```python
from build123d import *

# Parameters (mm, degrees)
F1_R     = 11.980735
F2_DEPTH = 23
F0_R     = 28.575
F0_R_2   = 2.54
F3_DEPTH = 4


with BuildPart() as f2:
    # F1 (on Front) → F2 (new body)
    with BuildSketch(Plane.XZ):
        with Locations((-0.001662, -0.397164)):
            Circle(F1_R)
        with BuildLine():
            add(Edge.make_bspline(
                [(2.011906, 7.609146), (2.011906, 7.809895), (2.011906, 8.211393), (2.011906, 8.813639), (2.011906, 9.215137), (2.011906, 9.415886)],
                knots=[0, 0, 0, 0, 0.602247, 1.204493, 1.80674, 1.80674, 1.80674, 1.80674], degree=3))
            ThreePointArc((2.011906, 7.609146), (4.126154, 6.752423), (5.925221, 5.349793))
            add(Edge.make_bspline(
                [(7.489904, 6.253163), (7.316434, 6.15301), (6.969194, 5.952531), (6.447633, 5.651408), (6.099543, 5.450437), (5.925221, 5.349793)],
                knots=[0, 0, 0, 0, 0.600918, 1.202873, 1.80674, 1.80674, 1.80674, 1.80674], degree=3))
            ThreePointArc((7.489904, 6.253163), (8.673752, 4.611589), (9.503473, 2.765559))
            add(Edge.make_bspline(
                [(7.93879, 1.862189), (8.113111, 1.962834), (8.461202, 2.163804), (8.982763, 2.464927), (9.330002, 2.665406), (9.503473, 2.765559)],
                knots=[0, 0, 0, 0, 0.603867, 1.205822, 1.80674, 1.80674, 1.80674, 1.80674], degree=3))
            ThreePointArc((7.93879, 1.862189), (8.25397, -0.397164), (7.93879, -2.656517))
            add(Edge.make_bspline(
                [(9.503473, -3.559887), (9.330002, -3.459734), (8.982763, -3.259255), (8.461202, -2.958132), (8.113111, -2.757162), (7.93879, -2.656517)],
                knots=[0, 0, 0, 0, 0.600918, 1.202873, 1.80674, 1.80674, 1.80674, 1.80674], degree=3))
            ThreePointArc((9.503473, -3.559887), (8.673752, -5.405917), (7.489904, -7.047491))
            add(Edge.make_bspline(
                [(5.925221, -6.144121), (6.099543, -6.244765), (6.447633, -6.445736), (6.969194, -6.746859), (7.316434, -6.947338), (7.489904, -7.047491)],
                knots=[0, 0, 0, 0, 0.603867, 1.205822, 1.80674, 1.80674, 1.80674, 1.80674], degree=3))
            ThreePointArc((5.925221, -6.144121), (4.126154, -7.546751), (2.011906, -8.403474))
            add(Edge.make_bspline(
                [(2.011906, -10.210214), (2.011906, -10.009465), (2.011906, -9.607967), (2.011906, -9.005721), (2.011906, -8.604223), (2.011906, -8.403474)],
                knots=[0, 0, 0, 0, 0.602247, 1.204493, 1.80674, 1.80674, 1.80674, 1.80674], degree=3))
            ThreePointArc((2.011906, -10.210214), (-0.001662, -10.414669), (-2.015231, -10.210214))
            add(Edge.make_bspline(
                [(-2.015231, -8.403474), (-2.015231, -8.604223), (-2.015231, -9.005721), (-2.015231, -9.607967), (-2.015231, -10.009465), (-2.015231, -10.210214)],
                knots=[0, 0, 0, 0, 0.602247, 1.204493, 1.80674, 1.80674, 1.80674, 1.80674], degree=3))
            ThreePointArc((-2.015231, -8.403474), (-4.129479, -7.546751), (-5.928546, -6.144121))
            add(Edge.make_bspline(
                [(-7.493228, -7.047491), (-7.319758, -6.947338), (-6.972519, -6.746859), (-6.450958, -6.445736), (-6.102867, -6.244765), (-5.928546, -6.144121)],
                knots=[0, 0, 0, 0, 0.600918, 1.202873, 1.80674, 1.80674, 1.80674, 1.80674], degree=3))
            ThreePointArc((-7.493228, -7.047491), (-8.677076, -5.405917), (-9.506797, -3.559887))
            add(Edge.make_bspline(
                [(-7.942115, -2.656517), (-8.116436, -2.757162), (-8.464527, -2.958132), (-8.986088, -3.259255), (-9.333327, -3.459734), (-9.506797, -3.559887)],
                knots=[0, 0, 0, 0, 0.603867, 1.205822, 1.80674, 1.80674, 1.80674, 1.80674], degree=3))
            ThreePointArc((-7.942115, -2.656517), (-8.257295, -0.397164), (-7.942115, 1.862189))
            add(Edge.make_bspline(
                [(-9.506797, 2.765559), (-9.333327, 2.665406), (-8.986088, 2.464927), (-8.464527, 2.163804), (-8.116436, 1.962834), (-7.942115, 1.862189)],
                knots=[0, 0, 0, 0, 0.600918, 1.202873, 1.80674, 1.80674, 1.80674, 1.80674], degree=3))
            ThreePointArc((-9.506797, 2.765559), (-8.677076, 4.611589), (-7.493228, 6.253163))
            add(Edge.make_bspline(
                [(-5.928546, 5.349793), (-6.102867, 5.450437), (-6.450958, 5.651408), (-6.972519, 5.952531), (-7.319758, 6.15301), (-7.493228, 6.253163)],
                knots=[0, 0, 0, 0, 0.603867, 1.205822, 1.80674, 1.80674, 1.80674, 1.80674], degree=3))
            ThreePointArc((-5.928546, 5.349793), (-4.129479, 6.752423), (-2.015231, 7.609146))
            add(Edge.make_bspline(
                [(-2.015231, 9.415886), (-2.015231, 9.215137), (-2.015231, 8.813639), (-2.015231, 8.211393), (-2.015231, 7.809895), (-2.015231, 7.609146)],
                knots=[0, 0, 0, 0, 0.602247, 1.204493, 1.80674, 1.80674, 1.80674, 1.80674], degree=3))
            ThreePointArc((-2.015231, 9.415886), (-0.001662, 9.620341), (2.011906, 9.415886))
        make_face(mode=Mode.SUBTRACT)
    extrude(amount=F2_DEPTH)

    # F0 (on Front) → F3 (join)
    with BuildSketch(Plane.XZ):
        Circle(F0_R)
        with Locations((-12.036908, -20.535689)):
            Circle(F0_R_2, mode=Mode.SUBTRACT)
        with Locations((11.767376, -20.535689)):
            Circle(F0_R_2, mode=Mode.SUBTRACT)
        with Locations((-23.8, 0)):
            Circle(F0_R_2, mode=Mode.SUBTRACT)
        with Locations((-11.988438, 20.600075)):
            Circle(F0_R_2, mode=Mode.SUBTRACT)
        with Locations((23.8, 0)):
            Circle(F0_R_2, mode=Mode.SUBTRACT)
        with Locations((11.78722, 20.636372)):
            Circle(F0_R_2, mode=Mode.SUBTRACT)
    extrude(amount=F3_DEPTH)


solid = f2.part
```
Work out the finished part from the listing and answer in its coordinate system (mm). A direction names the side the tool comes from. Coordinates: 2 decimals unless noted, no trailing zeros. Order: outer loops, then holes, each group sorted by start corner. A loop starts at its lowest first (then second) coordinate and runs counter-clockwise, first axis right, second up. Notation, with made-up numbers: (42, -37.75) - (98, -37.75) arc R21 cw to (98, -6.75) - close; hole circle Ø11 at (48.5, 75.5). An arc over 180 degrees is marked (long way). Answer as a JSON object with one key per item and string values.
1. The mould has two halves that part along Z. Classify faces 1 (the face through (0, 0, 0)), 2 (the face through (-28.547, -1.972, 1.256)), 3 (the face through (-9.566, -1.972, 21.363)): +Z half, -Z half, draft (parallel to the pull), parting line (faces both ways), or undercut.
Output values:
{"face 1": "draft", "face 2": "parting line", "face 3": "undercut"}
2. Consider line 1 (Z direction, x = 23.8, y = -2.55); line 2 (Y direction, x = 16.5, z = 22.5); line 3 (X direction, y = -18.75, z = 2). Determine where each line is inside the solid, lowest interval first.
Output values:
{"line 1": "z = -15.81 to -2.54, 2.54 to 15.81", "line 2": "y = -4 to 0", "line 3": "x = -11.74 to -8.18, 8.18 to 11.74"}
3. A tool of negligible diameter and unlimited length cuts with its end or side. For faces 4 (the face through (4.154, -13.367, -7.531)), 5 (the face through (-14.053, -1.972, -22.081)), from which of +Z, -Z, +X, -X, +Y, -Y can it reach the whole face along a straight path? Write none if from no direction.
Output values:
{"face 4": "-Y", "face 5": "+Y, -Y"}
4. Each of these flat-tipped pins is pushed along its axis until it touches: P1, Ø4.5, axis at x = 11.77, z = -20.54, coming from the +Y side; P2, Ø12, axis at x = -21.5, y = -9, coming from the +Z side; P3, Ø4, axis at x = 13.5, z = 18.5, coming from the +Y side; P4, Ø8, axis at x = -3.5, y = -6.5, coming from the -Z side. Where does it stop, or does it pass through?
Output values:
{"P1": "passes through", "P2": "stops at z = 22.04", "P3": "stops at y = 0", "P4": "stops at z = -28.57"}
5. Find section A-A on x = 23.8. Determine the outline of the cut face in (y, z), plus the area to 3 significant figures.
Output values:
{"outline": "(-4, -15.81) - (0, -15.81) - (0, -2.54) - (-4, -2.54) - close; (-4, 2.54) - (0, 2.54) - (0, 15.81) - (-4, 15.81) - close", "area": "106 mm²"}
6. Find section B-B on x = 0. Determine the outline of the cut face in (y, z) (3 decimals), plus the area to 3 significant figures.
Output values:
{"outline": "(-23, -12.378) - (-4, -12.378) - (-4, -28.575) - (0, -28.575) - (0, 28.575) - (-4, 28.575) - (-4, 11.584) - (-23, 11.584) - (-23, 9.62) - (-4, 9.62) - (-4, -10.415) - (-23, -10.415) - close", "area": "303 mm²"}
